Read the model definition and answer for the solid it produces. Units are mm, in the model's axes. Face numbers are marked on the shaded views. A direction names the side the tool comes from. Give positions to 0.01 mm unless a question says otherwise; leave off trailing zeros. Loops run counter-clockwise (first coordinate to the right, second up) from the corner with the lowest first, then second, coordinate; pieces in that order, holes last. Notation, with made-up numbers: (84, -0.5) -> (118, -0.5) arc R29 cw to (118, 31.5) -> close; hole circle Ø7 at (-24, -9.75). An arc over 180 degrees is marked (long way). Return JSON: item names as keys, results as strings. Group by question number.
from build123d import *

# Parameters (mm, degrees)
F1_DEPTH = 63.5
F0_W     = 25.4
F0_H     = 19.05
F0_H_2   = 4.7498
F0_H_3   = 4.7752
F2_DEPTH = 25.4
F4_DEPTH = 3.175
F5_R     = 12.7


with BuildPart() as f1:
    # F0 (on Front) → F1 (new body, symmetric)
    with BuildSketch(Plane.XZ):
        Polygon((41.275, -9.525), (41.275, 9.525), (22.225, 9.525), (-41.275, 9.525), (-41.275, -9.525), align=None)
    extrude(amount=F1_DEPTH, both=True)

    # F0 (on Front) → F2 (join, symmetric)
    with BuildSketch(Plane.XZ):
        with BuildLine():
            Line((22.225, 9.525), (41.275, 9.525))
            Line((41.275, 9.525), (41.275, 27.0002))
            ThreePointArc((41.275, 27.0002), (45.9246798487, 38.2255201513), (57.15, 42.8752))
            Line((57.15, 42.8752), (60.325, 42.8752))
            Line((60.325, 42.8752), (60.325, 61.9252))
            Line((60.325, 61.9252), (57.15, 61.9252))
            add(Edge.make_bspline(
                [(55.8906627655, 61.9024878151), (56.3095920905, 61.9105285601), (56.7293746708, 61.9180961221), (57.15, 61.9252)],
                knots=[110.683860184, 110.683860184, 110.683860184, 110.683860184, 111.5045361635, 111.5045361635, 111.5045361635, 111.5045361635], degree=3))
            ThreePointArc((55.8906627655, 61.9024878151), (32.0129956248, 51.2465736679), (22.225, 27.0002))
            Line((22.225, 27.0002), (22.225, 9.525))
        make_face()
        with Locations((73.025, 52.4002)):
            Rectangle(F0_W, F0_H)
        with Locations((73.025, 64.3001)):
            Rectangle(F0_W, F0_H_2)
        with Locations((73.025, 40.4876)):
            Rectangle(F0_W, F0_H_3)
    extrude(amount=F2_DEPTH, both=True)

    # F0 (on Front) → F3 (revolve)
    with BuildSketch(Plane.XZ):
        Polygon((85.725, 61.9252), (85.725, 42.8752), (85.725, 38.1), (111.125, 38.1), (111.125, 66.675), (85.725, 66.675), align=None)
    revolve(axis=Axis((85.725, 0, 52.3875), (0, 0, 1)))

    # F0 (on Front) → F4 (join, symmetric)
    with BuildSketch(Plane.XZ):
        with BuildLine():
            Line((-41.275, 9.525), (22.225, 9.525))
            Line((22.225, 9.525), (22.225, 27.0002))
            ThreePointArc((22.225, 27.0002), (32.0129956248, 51.2465736679), (55.8906627655, 61.9024878151))
            add(Edge.make_bspline(
                [(-41.275, 9.525), (-41.5901642884, 51.126542611), (-0.6099732885, 60.8180394914), (55.8906627655, 61.9024878151)],
                knots=[0, 0, 0, 0, 110.683860184, 110.683860184, 110.683860184, 110.683860184], degree=3))
        make_face()
    extrude(amount=F4_DEPTH, both=True)

    # F5
    f5_edges = [f1.edges().sort_by_distance(p)[0] for p in [
        (85.725, 25.4, 52.3875),
        (73.025, 25.4, 66.675),
        (73.025, -25.4, 66.675),
        (111.125, 0, 66.675),
    ]]
    fillet(f5_edges, radius=F5_R)


solid = f1.part
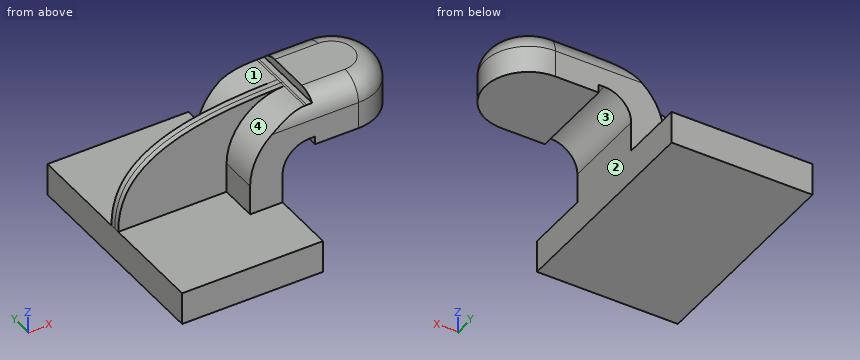
1. Flat-ended cylindrical pins translate along their axes: pin 1 Ø1.6 at (x, y) = (59, -9.5) entering from -Z; pin 2 Ø4 at (x, z) = (2, 29.5) entering from +Y (3 decimals); pin 3 Ø22 at (x, z) = (58, 37) entering from +Y. Find the tip coordinate at first contact, or state that the pin passes through.
2. Which of the six approach directions +Z, -Z, +X, -X, +Y, -Y give full straight-line access (tool end or side, diameter ignored) to the marked faces 1, 2, 3 and 4?
3. Section A-A on y = 52 is taken. Determine the outline of the cut face in (x, z) (3 decimals), then the cut area to 3 significant figures.
4. Section B-B on z = -4 is taken. Determine the outline of the cut face in (x, y) (3 decimals).
5. Straight lines are drawn through the part: line 1 (Z direction, x = -2, y = 36) (3 decimals); line 2 (Y direction, x = -17, z = 37) (3 decimals); line 3 (X direction, y = 19, z = -2.5) (3 decimals). For each, find the intervals that lie inside material, in ascending order. Write a range as from..to.
Completed:
{
 "1": {"pin 1": "stops at z = 42.88", "pin 2": "stops at y = 3.175", "pin 3": "stops at y = 25.4"},
 "2": {"face 1": "+Z, -X, +Y", "face 2": "-Z, +X, +Y, -Y", "face 3": "-Z, +Y, -Y", "face 4": "+Z, -X, -Y"},
 "3": {"outline": "(-41.275, -9.525) -> (41.275, -9.525) -> (41.275, 9.525) -> (-41.275, 9.525) -> close", "area": "1,570 mm²"},
 "4": {"outline": "(-41.275, -63.5) -> (41.275, -63.5) -> (41.275, 63.5) -> (-41.275, 63.5) -> close"},
 "5": {"line 1": "z = -9.525..9.525", "line 2": "y = -3.175..3.175", "line 3": "x = -41.275..41.275"}
}
